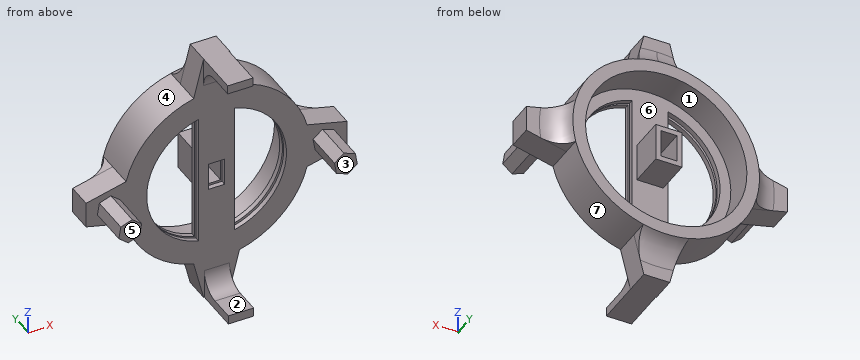
```python
from build123d import *

# Parameters (mm, degrees)
SKETCH4_R                = 17
BOSS_EXTRUDE3_DEPTH      = 6
SHELL4_T                 = 0.5
SKETCH5_W                = 3.2
SKETCH5_H                = 5.5
BOSS_EXTRUDE4_DEPTH      = 8
SHELL5_T                 = 1
BOSS_EXTRUDE6_DEPTH      = 3.5
BOSS_EXTRUDE6_DEPTH_BACK = 1.5
SKETCH7_W                = 5
SKETCH7_H                = 1.75
BOSS_EXTRUDE7_DEPTH      = 9
FILLET3_R                = 5
CUT_EXTRUDE1_DEPTH       = 5
SKETCH13_W               = 3.166032567
SKETCH13_H               = 5.463514234
CUT_EXTRUDE2_DEPTH       = 5
FILLET4_R                = 4
BOSS_EXTRUDE8_DEPTH      = 8


with BuildPart() as part:
    # Sketch4 → Boss-Extrude3 (new body)
    with BuildSketch(Plane(origin=(0, 0, 0), x_dir=(1, 0, 0), z_dir=(0, 1, 0))):
        with Locations(Location((0, -46.79046007, 0), (0, 0, 270))):
            Circle(SKETCH4_R)
    extrude(amount=BOSS_EXTRUDE3_DEPTH)

    # Shell4
    shell4_openings = [part.faces().sort_by_distance(p)[0] for p in [
        (0, 6, 46.79046007),
    ]]
    offset(amount=SHELL4_T, openings=shell4_openings, kind=Kind.INTERSECTION)

    # Sketch5 → Boss-Extrude4 (add)
    with BuildSketch(Plane(origin=(0, 0, 0), x_dir=(1, 0, 0), z_dir=(0, 1, 0))):
        with Locations((0, -46.79046007)):
            Rectangle(SKETCH5_W, SKETCH5_H)
    extrude(amount=BOSS_EXTRUDE4_DEPTH)

    # Shell5
    shell5_openings = [part.faces().sort_by_distance(p)[0] for p in [
        (0, 8, 46.79046007),
    ]]
    offset(amount=SHELL5_T, openings=shell5_openings, kind=Kind.INTERSECTION)

    # Sketch6 → Boss-Extrude6 (add, two sides: drawn at the far end of the back side and taken through both)
    with BuildSketch(Plane(origin=(0, 0, 0), x_dir=(1, 0, 0), z_dir=(0, 1, 0)).offset(-BOSS_EXTRUDE6_DEPTH_BACK)):
        with BuildLine():
            Line((-2.565219646, -72.659781842), (2.565219646, -72.659781842))
            Line((2.565219646, -72.659781842), (4.531236217, -64.726956337))
            ThreePointArc((4.531236217, -64.726956337), (0, -65.29046007), (-4.531236217, -64.726956337))
            Line((-4.531236217, -64.726956337), (-2.565219646, -72.659781842))
        make_face()
        with BuildLine():
            Line((-25.869321772, -44.225240424), (-17.936496267, -42.259223853))
            ThreePointArc((-17.936496267, -42.259223853), (-18.5, -46.79046007), (-17.936496267, -51.321696288))
            Line((-17.936496267, -51.321696288), (-25.869321772, -49.355679717))
            Line((-25.869321772, -49.355679717), (-25.869321772, -44.225240424))
        make_face()
        with BuildLine():
            Line((2.565219646, -20.921138298), (4.531236217, -28.853963803))
            ThreePointArc((4.531236217, -28.853963803), (0, -28.29046007), (-4.531236217, -28.853963803))
            Line((-4.531236217, -28.853963803), (-2.565219646, -20.921138298))
            Line((-2.565219646, -20.921138298), (2.565219646, -20.921138298))
        make_face()
        with BuildLine():
            Line((25.869321772, -49.355679717), (17.936496267, -51.321696288))
            ThreePointArc((17.936496267, -51.321696288), (18.5, -46.79046007), (17.936496267, -42.259223853))
            Line((17.936496267, -42.259223853), (25.869321772, -44.225240424))
            Line((25.869321772, -44.225240424), (25.869321772, -49.355679717))
        make_face()
    extrude(amount=BOSS_EXTRUDE6_DEPTH + BOSS_EXTRUDE6_DEPTH_BACK)

    # Sketch7 → Boss-Extrude7 (add)
    with BuildSketch(Plane(origin=(0, -1.5, 0), x_dir=(-1, 0, 0), z_dir=(0, -1, 0))):
        with Locations((0.065219646, -71.784781842)):
            Rectangle(SKETCH7_W, SKETCH7_H)
        with Locations((-0.065219646, -21.796138298)):
            Rectangle(SKETCH7_W, SKETCH7_H)
    extrude(amount=BOSS_EXTRUDE7_DEPTH)

    # Fillet3
    # the kernel refuses this fillet: 5 mm, written as the material it adds along each edge
    with BuildSketch(Plane(origin=(0, 3.5, 46.79046007), x_dir=(-0.6278344871312538, 0, -0.7783468743231616), z_dir=(0.7783468743231616, 0, -0.6278344871312538))) as fillet3_piece_1_section:
        with BuildLine():
            CenterArc((23.269696007, 5), FILLET3_R, 197.457603124, 72.542396876)
            Line((23.269696007, 0), (23.269696007, -0.1))
            Line((23.269696007, -0.1), (18.5, -0.1))
            Line((18.5, -0.1), (18.4, 0))
            ThreePointArc((18.4, 0), (18.4, 1.75), (18.40460608, 3.47))
            Line((18.40460608, 3.47), (18.5, 3.5))
        make_face()
    fillet3_piece_1 = revolve(axis=Axis((0, 3.5, 46.79046007), (0, 1, 0)), revolution_arc=102.218929963, mode=Mode.PRIVATE)
    fillet3_piece_1 = split(fillet3_piece_1, bisect_by=Plane(origin=(-20.380505818, 4.426759582, 42.864930265), z_dir=(0.24055555302697984, 0, 0.9706353722731745)), keep=Keep.TOP, mode=Mode.PRIVATE)
    fillet3_piece_1 = split(fillet3_piece_1, bisect_by=Plane(origin=(-20.380505744, 4.426759582, 50.715989893), z_dir=(0.24055555302697348, 0, -0.9706353722731761)), keep=Keep.TOP, mode=Mode.PRIVATE)
    add(fillet3_piece_1)
    with BuildSketch(Plane(origin=(0, 3.5, 46.79046007), x_dir=(0.7783347748418207, 0, 0.6278494869568123), z_dir=(0.6278494869568123, 0, -0.7783347748418207))) as fillet3_piece_2_section:
        with BuildLine():
            CenterArc((23.269696007, -5), FILLET3_R, 90, 72.542396876)
            Line((23.269696007, 0), (23.269696007, 0.1))
            Line((23.269696007, 0.1), (18.5, 0.1))
            Line((18.5, 0.1), (18.4, 0))
            ThreePointArc((18.4, 0), (18.4, -1.75), (18.40460608, -3.47))
            Line((18.40460608, -3.47), (18.5, -3.5))
        make_face()
    fillet3_piece_2 = revolve(axis=Axis((0, 3.5, 46.79046007), (0, -1, 0)), revolution_arc=51.108360804, mode=Mode.PRIVATE)
    fillet3_piece_2 = split(fillet3_piece_2, bisect_by=Plane(origin=(4.048850537, 4.426759722, 66.673369956), z_dir=(-0.970635372273176, 0, -0.24055555302697343)), keep=Keep.TOP, mode=Mode.PRIVATE)
    add(fillet3_piece_2)
    with BuildSketch(Plane(origin=(0, 3.5, 46.79046007), x_dir=(0.7783468743230912, 0, -0.6278344871313409), z_dir=(0.6278344871313409, 0, 0.7783468743230912))) as fillet3_piece_3_section:
        with BuildLine():
            CenterArc((23.269696007, 5), FILLET3_R, 197.457603124, 72.542396876)
            Line((23.269696007, 0), (23.269696007, -0.1))
            Line((23.269696007, -0.1), (18.5, -0.1))
            Line((18.5, -0.1), (18.4, 0))
            ThreePointArc((18.4, 0), (18.4, 1.75), (18.40460608, 3.47))
            Line((18.40460608, 3.47), (18.5, 3.5))
        make_face()
    fillet3_piece_3 = revolve(axis=Axis((0, 3.5, 46.79046007), (0, 1, 0)), revolution_arc=102.218929963, mode=Mode.PRIVATE)
    fillet3_piece_3 = split(fillet3_piece_3, bisect_by=Plane(origin=(3.925529805, 4.426759582, 26.409954252), z_dir=(-0.9706353722731743, 0, 0.24055555302698087)), keep=Keep.TOP, mode=Mode.PRIVATE)
    fillet3_piece_3 = split(fillet3_piece_3, bisect_by=Plane(origin=(-3.925529823, 4.426759582, 26.409954326), z_dir=(0.9706353722731764, 0, 0.2405555530269717)), keep=Keep.TOP, mode=Mode.PRIVATE)
    add(fillet3_piece_3)
    with BuildSketch(Plane(origin=(0, 3.5, 46.79046007), x_dir=(0.6278344871312218, 0, 0.7783468743231875), z_dir=(-0.7783468743231875, 0, 0.6278344871312218))) as fillet3_piece_4_section:
        with BuildLine():
            CenterArc((23.269696007, 5), FILLET3_R, 197.457603124, 72.542396876)
            Line((23.269696007, 0), (23.269696007, -0.1))
            Line((23.269696007, -0.1), (18.5, -0.1))
            Line((18.5, -0.1), (18.4, 0))
            ThreePointArc((18.4, 0), (18.4, 1.75), (18.40460608, 3.47))
            Line((18.40460608, 3.47), (18.5, 3.5))
        make_face()
    fillet3_piece_4 = revolve(axis=Axis((0, 3.5, 46.79046007), (0, 1, 0)), revolution_arc=102.218929963, mode=Mode.PRIVATE)
    fillet3_piece_4 = split(fillet3_piece_4, bisect_by=Plane(origin=(20.380505818, 4.426759582, 50.715989875), z_dir=(-0.24055555302698112, 0, -0.9706353722731741)), keep=Keep.TOP, mode=Mode.PRIVATE)
    fillet3_piece_4 = split(fillet3_piece_4, bisect_by=Plane(origin=(20.380505744, 4.426759582, 42.864930247), z_dir=(-0.24055555302697304, 0, 0.9706353722731761)), keep=Keep.TOP, mode=Mode.PRIVATE)
    add(fillet3_piece_4)
    with BuildSketch(Plane(origin=(0, 3.5, 46.79046007), x_dir=(0, 0, 1), z_dir=(1, 0, 0))) as fillet3_piece_5_section:
        with BuildLine():
            CenterArc((23.269696007, -5), FILLET3_R, 90, 72.542396876)
            Line((23.269696007, 0), (23.269696007, 0.1))
            Line((23.269696007, 0.1), (18.5, 0.1))
            Line((18.5, 0.1), (18.4, 0))
            ThreePointArc((18.4, 0), (18.4, -1.75), (18.40460608, -3.47))
            Line((18.40460608, -3.47), (18.5, -3.5))
        make_face()
    fillet3_piece_5 = revolve(axis=Axis((0, 3.5, 46.79046007), (0, -1, 0)), revolution_arc=51.108360804, mode=Mode.PRIVATE)
    fillet3_piece_5 = split(fillet3_piece_5, bisect_by=Plane(origin=(-4.04885046, 4.426759578, 66.673370268), z_dir=(0.9706353722731745, 0, -0.24055555302697917)), keep=Keep.TOP, mode=Mode.PRIVATE)
    add(fillet3_piece_5)

    # Sketch11 → Cut-Extrude1 (cut)
    with BuildSketch(Plane(origin=(0, 1, 0), x_dir=(1, 0, 0), z_dir=(0, 1, 0))):
        with BuildLine():
            Line((-3.585868376, -59.921550203), (-3.585868376, -33.501237191))
            ThreePointArc((-3.585868376, -33.501237191), (-13.861572731, -46.711393697), (-3.585868376, -59.921550203))
        make_face()
        with BuildLine():
            Line((3.585868376, -59.921550203), (3.585868376, -33.501237191))
            ThreePointArc((3.585868376, -33.501237191), (13.861572731, -46.711393697), (3.585868376, -59.921550203))
        make_face()
    extrude(amount=-CUT_EXTRUDE1_DEPTH, mode=Mode.SUBTRACT)

    # Sketch13 → Cut-Extrude2 (cut)
    with BuildSketch(Plane(origin=(0, -0.5, 0), x_dir=(1, 0, 0), z_dir=(0, 1, 0))):
        with Locations((0.016983716, -46.772217187)):
            Rectangle(SKETCH13_W, SKETCH13_H)
    extrude(amount=-CUT_EXTRUDE2_DEPTH, mode=Mode.SUBTRACT)

    # Fillet4
    fillet4_edges = [part.edges().sort_by_distance(p)[0] for p in [
        (0.065219646, -1.5, 22.671138298),
        (-0.065219646, -1.5, 70.909781842),
    ]]
    fillet(fillet4_edges, radius=FILLET4_R)

    # Sketch16 → Boss-Extrude8 (add)
    with BuildSketch(Plane(origin=(0, -1.5, 0), x_dir=(-1, 0, 0), z_dir=(0, -1, 0))):
        Polygon((19.095115037, -47.769177252), (20.96203058, -49.305079029), (23.225618307, -48.456233631), (23.622290493, -46.071486456), (21.75537495, -44.535584679), (19.491787223, -45.384430077), align=None)
        Polygon((-19.525754656, -45.384430077), (-19.12908247, -47.769177252), (-20.995998013, -49.305079029), (-23.25958574, -48.456233631), (-23.656257926, -46.071486456), (-21.789342383, -44.535584679), align=None)
    extrude(amount=BOSS_EXTRUDE8_DEPTH)


solid = part.part
```
Build history of the part. All positions in model axes, mm. Face numbers are marked on the shaded views. A direction names the side the tool comes from. Round coordinates to 2 decimals unless told otherwise and drop trailing zeros. Write each loop counter-clockwise with the first axis right and the second up, starting at its lowest first coordinate (ties: lowest second). Pieces come first, ordered by that corner, then holes.
1) Pin check, flat tips, straight feed: pin 1 (10.5 mm diameter, centred on x = -0.5, z = 51, fed in from -Y); pin 2 (2.5 mm diameter, centred on x = 21.5, z = 47.5, fed in from -Y); pin 3 (8 mm diameter, centred on x = 1.5, z = 45.5, fed in from +Y); pin 4 (3 mm diameter, centred on y = 5.5, z = 46.5, fed in from +X). Stop position of each tip, or through.
2) Band-saw the part on A-A, the plane y = 5.25. List the corners of the cut face in (x, z).
3) Drill centre lines: probe 1 along Y at (x, z) = (15.5, 50); probe 2 along Z at (x, y) = (-13, 1.25); probe 3 along Y at (x, z) = (15, 56). Where is each one in solid material? Low to high.
4) Band-saw the part on C-C, the plane z = 37. Give the number of separate pieces and of enclosed holes in the cut face, and give its area (3 significant figures).
5) 3-axis set-ups, long thin cutter, end or side, ignore diameter. For the marked faces 1, 2 and 3: which of +Z, -Z, +X, -X, +Y, -Y reach the whole face in a straight line?
6) Mould opens along X. For the marked faces 4, 5, 6 and 7 say: +X half, -X half, draft (parallel to the pull), parting line (faces both ways), or undercut.
7) Band-saw the part on B-B, the plane x = -6. List the corners of the cut face in (y, z), and give its area (3 significant figures).
Ans:
1. pin 1: stops at y = -1.5
1. pin 2: stops at y = -9.5
1. pin 3: stops at y = 8
1. pin 4: stops at x = 21.09
2. outline: (-19, 42.52) - (-17.94, 42.26) arc R18.5 ccw to (-4.53, 28.85) - (-4.27, 27.79) arc R19.47 ccw to (4.27, 27.79) - (4.53, 28.85) arc R18.5 ccw to (17.94, 42.26) - (19, 42.52) arc R19.47 ccw to (19, 51.06) - (17.94, 51.32) arc R18.5 ccw to (4.53, 64.73) - (4.27, 65.79) arc R19.47 ccw to (-4.27, 65.79) - (-4.53, 64.73) arc R18.5 ccw to (-17.94, 51.32) - (-19, 51.06) arc R19.47 ccw to start; circle Ø34 at (0, 46.79); (-2.6, 43.04) - (2.6, 43.04) - (2.6, 50.54) - (-2.6, 50.54) - close; hole circle Ø35 at (0, 46.79); hole circle Ø32 at (0, 46.79); hole (-1.6, 44.04) - (1.6, 44.04) - (1.6, 49.54) - (-1.6, 49.54) - close
3. probe 1: y = -1.5 to -0.5, 0 to 1
3. probe 2: z = 33.63 to 35.08, 35.84 to 37.46, 56.12 to 57.74, 58.51 to 59.95
3. probe 3: y = -1.5 to 7
4. separate pieces: 4
4. enclosed holes: 0
4. area: 68.4 mm2
5. face 1: +Y
5. face 2: +X, -X, -Y
5. face 3: +Z, -Z, +X, -X, -Y
6. face 4: -X half
6. face 5: draft
6. face 6: undercut
6. face 7: +X half
7. outline: (-1.5, 29.29) - (7, 29.29) - (7, 31.96) - (1, 31.96) - (1, 34.36) - (0, 34.36) - (0, 30.88) - (6, 30.88) - (6, 30.35) - (-0.5, 30.35) - (-0.5, 34.36) - (-1.5, 34.36) - close; (-1.5, 59.06) - (-0.5, 59.06) - (-0.5, 63.23) - (6, 63.23) - (6, 62.7) - (0, 62.7) - (0, 59.06) - (1, 59.06) - (1, 61.62) - (7, 61.62) - (7, 64.29) - (-1.5, 64.29) - close
7. area: 47.3 mm2
